Geometry: final body of the model. Coordinates: model frame, mm. A direction names the side the tool comes from. Give positions to 0.01 mm unless a question says otherwise; leave off trailing zeros. Order: outer loops, then holes, each group sorted by start corner. A loop starts at its lowest first (then second) coordinate and runs counter-clockwise, first axis right, second up. Notation, with made-up numbers: (32.25, -34.75) -> (41.25, -34.75) arc R20 cw to (41.25, -22.75) -> close; hole circle Ø11 at (-33, -31). An arc over 180 degrees is marked (long way). Answer in a Markdown table with one row per item. Add a question column.
Q1. Pull-direction query (Z, two-part tool) for faces 1 (the face through (55.682, 25, -113)), 2 (the face through (56, 35, -91)), 3 (the face through (56, 27, 16.767)); classes: +Z half, -Z half, draft (parallel to the pull), parting line (faces both ways), or undercut.
Q2. Cut plane C-C on x = 7. Return the cut outline in (y, z).
Q3. Cut plane A-A on y = 15.25. Count the separate pieces of the cut face and the enclosed holes in it, and give its area (3 significant figures).
Q4. Cut plane B-B on x = 29. Return the cut outline in (y, z).
Q5. Contact query for flat-ended pins moving along their axis: P1, Ø11.5, axis at x = 55.5, z = -47.5, coming from the +Y side; P2, Ø3, axis at y = 24.75, z = -63.73, coming from the -X side; P3, Ø4.5, axis at x = 56, z = -42.5, coming from the -Y side; P4, Ø6, axis at y = 10, z = -42, coming from the -X side. Output: stop coordinate, or through.
Q6. Set-up query: faces 4 (the face through (25.682, 4, -51)), 5 (the face through (40, 20, -51)), 6 (the face through (-33.39, 10.09, -52.73)), 7 (the face through (45.682, 31, -11)), 8 (the face through (31.682, 32, -51)). Return all of +Z, -Z, +X, -X, +Y, -Y with unobstructed straight access to the full face (end or side cutting, diameter ignored); none if empty.
Q7. Line query: line 1 along Z through (x, y) = (55.5, 10); line 2 along X through (y, z) = (31.5, -28); line 3 along Z through (x, y) = (43, 19). Output: solid intervals per line, ascending. Write a range as from..to.
from build123d import *

# Parameters (mm, degrees)
BOSS_EXTRUDE1_DEPTH = 35
CUT_EXTRUDE1_REACH  = 163.307
SKETCH2_W           = 42
SKETCH2_H           = 21
SKETCH3_R           = 2
CUT_EXTRUDE2_DEPTH  = 10
FILLET1_R           = 20
CUT_EXTRUDE5_REACH  = 163.307
SKETCH6_W           = 42
SKETCH6_H           = 9
SKETCH7_R           = 2
CUT_EXTRUDE6_DEPTH  = 10
CUT_EXTRUDE7_DEPTH  = 9
SKETCH9_R           = 2
CUT_EXTRUDE8_DEPTH  = 10
CUT_EXTRUDE9_DEPTH  = 6
SKETCH11_R          = 2
CUT_EXTRUDE10_DEPTH = 9


with BuildPart() as part:
    # Sketch1 → Boss-Extrude1 (new body)
    with BuildSketch(Plane(origin=(0, 0, 0), x_dir=(1, 0, 0), z_dir=(0, 1, 0))):
        Polygon((-38.317617866, 43.23325062), (45.682382134, 43.23325062), (45.682382134, -16.76674938), (65.682382134, -16.76674938), (65.682382134, 118.23325062), (45.682382134, 118.23325062), (45.682382134, 58.23325062), (-38.317617866, 58.23325062), align=None)
    extrude(amount=BOSS_EXTRUDE1_DEPTH)

    # Sketch2 → Cut-Extrude1 (cut, up to next)
    with BuildSketch(Plane(origin=(65.682382134, 0, 0), x_dir=(0, 0, -1), z_dir=(1, 0, 0)), mode=Mode.PRIVATE) as cut_extrude1_sk1:
        with Locations((13.23325062, 19.5)):
            Rectangle(SKETCH2_W, SKETCH2_H)
    cut_extrude1_tool1 = extrude(cut_extrude1_sk1.sketch, amount=-CUT_EXTRUDE1_REACH, mode=Mode.PRIVATE) & part.part
    # Sketch2 → Cut-Extrude1 (cut, up to next)
    with BuildSketch(Plane(origin=(65.682382134, 0, 0), x_dir=(0, 0, -1), z_dir=(1, 0, 0)), mode=Mode.PRIVATE) as cut_extrude1_sk2:
        with Locations((88.23325062, 19.5)):
            Rectangle(SKETCH2_W, SKETCH2_H)
    cut_extrude1_tool2 = extrude(cut_extrude1_sk2.sketch, amount=-CUT_EXTRUDE1_REACH, mode=Mode.PRIVATE) & part.part
    add(cut_extrude1_tool1.solids().sort_by_distance((65.682382, 19.5, -13.233251))[0], mode=Mode.SUBTRACT)
    add(cut_extrude1_tool2.solids().sort_by_distance((65.682382, 19.5, -88.233251))[0], mode=Mode.SUBTRACT)

    # Sketch3 → Cut-Extrude2 (cut)
    with BuildSketch(Plane.ZY.offset(-45.682382134)):
        with Locations((11.26674938, 24.75)):
            Circle(SKETCH3_R)
        with Locations((11.26674938, 15.25)):
            Circle(SKETCH3_R)
        with Locations((-37.73325062, 24.75)):
            Circle(SKETCH3_R)
        with Locations((-37.73325062, 15.25)):
            Circle(SKETCH3_R)
        with Locations(Location((-112.73325062, 24.75, 0), (0, 0, 180))):
            Circle(SKETCH3_R)
        with Locations(Location((-112.73325062, 15.25, 0), (0, 0, 180))):
            Circle(SKETCH3_R)
        with Locations(Location((-63.73325062, 15.25, 0), (0, 0, 180))):
            Circle(SKETCH3_R)
        with Locations(Location((-63.73325062, 24.75, 0), (0, 0, 180))):
            Circle(SKETCH3_R)
    extrude(amount=-CUT_EXTRUDE2_DEPTH, mode=Mode.SUBTRACT)

    # Fillet1
    fillet1_edges = [part.edges().sort_by_distance(p)[0] for p in [
        (55.682382134, 0, -118.23325062),
        (55.682382134, 0, 16.76674938),
    ]]
    fillet(fillet1_edges, radius=FILLET1_R)

    # Sketch6 → Cut-Extrude5 (cut, up to next)
    with BuildSketch(Plane(origin=(65.682382134, 0, 0), x_dir=(0, 0, -1), z_dir=(1, 0, 0)), mode=Mode.PRIVATE) as cut_extrude5_sk1:
        with Locations((13.23325062, 4.5)):
            Rectangle(SKETCH6_W, SKETCH6_H)
    cut_extrude5_tool1 = extrude(cut_extrude5_sk1.sketch, amount=-CUT_EXTRUDE5_REACH, mode=Mode.PRIVATE) & part.part
    # Sketch6 → Cut-Extrude5 (cut, up to next)
    with BuildSketch(Plane(origin=(65.682382134, 0, 0), x_dir=(0, 0, -1), z_dir=(1, 0, 0)), mode=Mode.PRIVATE) as cut_extrude5_sk2:
        with Locations((88.23325062, 4.5)):
            Rectangle(SKETCH6_W, SKETCH6_H)
    cut_extrude5_tool2 = extrude(cut_extrude5_sk2.sketch, amount=-CUT_EXTRUDE5_REACH, mode=Mode.PRIVATE) & part.part
    add(cut_extrude5_tool1.solids().sort_by_distance((65.682382, 4.5, -13.233251))[0], mode=Mode.SUBTRACT)
    add(cut_extrude5_tool2.solids().sort_by_distance((65.682382, 4.5, -88.233251))[0], mode=Mode.SUBTRACT)

    # Sketch7 → Cut-Extrude6 (cut)
    with BuildSketch(Plane.ZY.offset(38.317617866)):
        with Locations((-50.73325062, 25)):
            Circle(SKETCH7_R)
        with Locations((-50.73325062, 10)):
            Circle(SKETCH7_R)
    extrude(amount=-CUT_EXTRUDE6_DEPTH, mode=Mode.SUBTRACT)

    # Sketch8 → Cut-Extrude7 (cut)
    with BuildSketch(Plane.XZ):
        Polygon((45.682382134, -67.23325062), (45.682382134, -58.23325062), (25.682382134, -58.23325062), (25.682382134, -43.23325062), (45.682382134, -43.23325062), (45.682382134, -34.23325062), (65.682382134, -34.23325062), (65.682382134, -67.23325062), align=None)
    extrude(amount=-CUT_EXTRUDE7_DEPTH, mode=Mode.SUBTRACT)

    # Sketch9 → Cut-Extrude8 (cut)
    with BuildSketch(Plane.XZ.offset(-9)):
        with Locations(Location((55.682382134, -42.23325062, 0), (0, 0, 270))):
            Circle(SKETCH9_R)
        with Locations(Location((55.682382134, -59.23325062, 0), (0, 0, 270))):
            Circle(SKETCH9_R)
        with Locations(Location((35.682382134, -50.73325062, 0), (0, 0, 270))):
            Circle(SKETCH9_R)
    extrude(amount=-CUT_EXTRUDE8_DEPTH, mode=Mode.SUBTRACT)

    # Sketch10 → Cut-Extrude9 (cut)
    with BuildSketch(Plane(origin=(0, 35, 0), x_dir=(1, 0, 0), z_dir=(0, 1, 0))):
        Polygon((45.682382134, 62.23325062), (65.682382134, 62.23325062), (65.682382134, 39.23325062), (45.682382134, 39.23325062), (45.682382134, 43.23325062), (31.682382134, 43.23325062), (31.682382134, 58.23325062), (45.682382134, 58.23325062), align=None)
    extrude(amount=-CUT_EXTRUDE9_DEPTH, mode=Mode.SUBTRACT)

    # Sketch11 → Cut-Extrude10 (cut)
    with BuildSketch(Plane(origin=(0, 29, 0), x_dir=(1, 0, 0), z_dir=(0, 1, 0))):
        with Locations(Location((55.682382134, 58.23325062, 0), (0, 0, 270))):
            Circle(SKETCH11_R)
        with Locations(Location((55.682382134, 43.23325062, 0), (0, 0, 270))):
            Circle(SKETCH11_R)
        with Locations(Location((39.682382134, 50.73325062, 0), (0, 0, 270))):
            Circle(SKETCH11_R)
    extrude(amount=-CUT_EXTRUDE10_DEPTH, mode=Mode.SUBTRACT)


solid = part.part
Completed:
| question | item | result |
|---|---|---|
| 1 | face 1 | undercut |
| 1 | face 2 | draft |
| 1 | face 3 | +Z half |
| 2 | outline | (0, -58.23) -> (35, -58.23) -> (35, -43.23) -> (0, -43.23) -> close |
| 3 | separate pieces | 3 |
| 3 | enclosed holes | 3 |
| 3 | area | 2,060 mm² |
| 4 | outline | (9, -58.23) -> (35, -58.23) -> (35, -43.23) -> (9, -43.23) -> close |
| 5 | P1 | stops at y = 29 |
| 5 | P2 | stops at x = 55.68 |
| 5 | P3 | stops at y = 9 |
| 5 | P4 | stops at x = -38.32 |
| 6 | face 4 | +Z, -Z, +X, -Y |
| 6 | face 5 | +Y |
| 6 | face 6 | -X |
| 6 | face 7 | +Z, -X, +Y, -Y |
| 6 | face 8 | +Z, -Z, +X, +Y |
| 7 | line 1 | z = -115.55..-109.23, -67.23..-61.22, -57.24..-44.22, -40.24..-34.23, 7.77..14.09 |
| 7 | line 2 | x = 45.68..65.68 |
| 7 | line 3 | z = -58.23..-43.23 |
